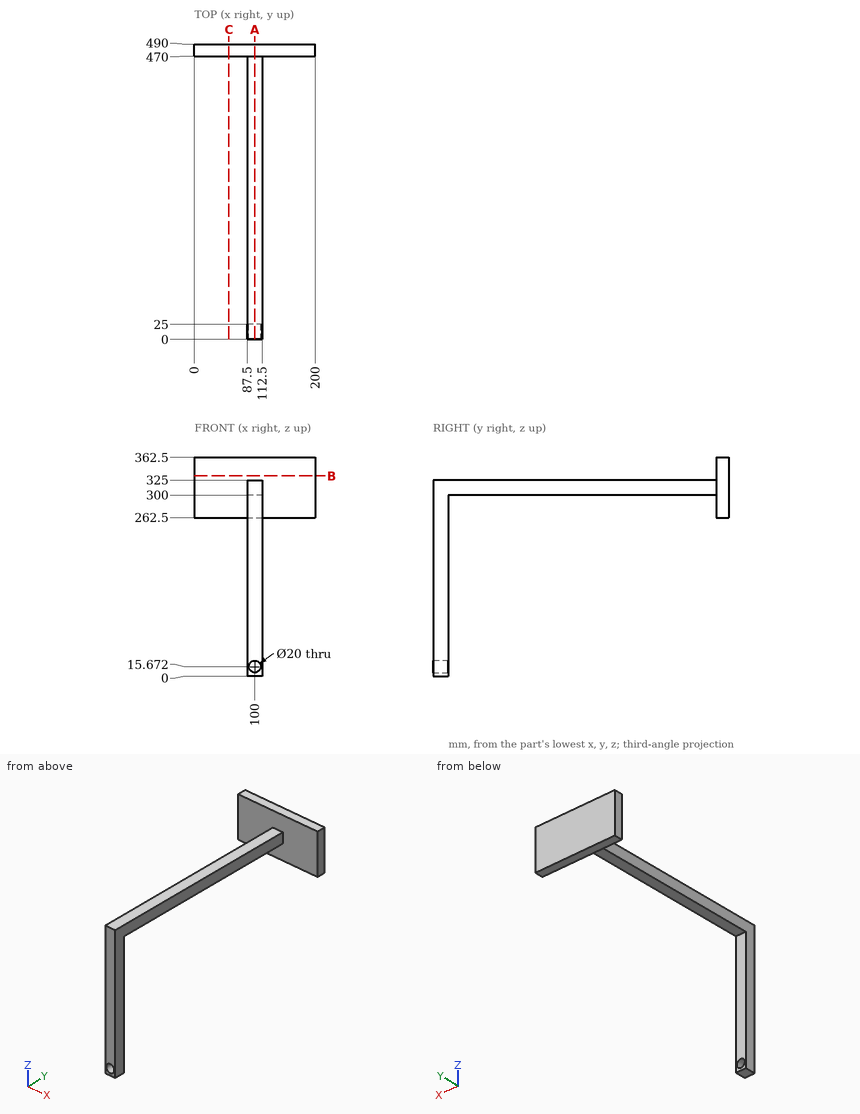
Geometry: see drawing. Coordinates: mm, zero at the bounding-box minimum. Coordinates: 2 decimals unless noted, no trailing zeros. Loops run counter-clockwise (first coordinate to the right, second up) from the corner with the lowest first, then second, coordinate; pieces in that order, holes last. Notation, with made-up numbers: (12.25, 46) -> (55.25, 46) arc R23 cw to (55.25, 82) -> close; hole circle Ø11 at (-31, 49). An arc over 180 degrees is marked (long way). Use a Markdown table: item, result.
1) Cut plane B-B (z = 332). Return the cut outline in (x, y), then the cut area to 3 significant figures.
Results found:
| item | result |
|---|---|
| outline | (0, 470) -> (200, 470) -> (200, 490) -> (0, 490) -> close |
| area | 4,000 mm2 |
2) Cut plane A-A (x = 100). Return the cut outline in (y, z), then the cut area to 4 significant figures.
Results found:
| item | result |
|---|---|
| outline | (0, 0) -> (25, 0) -> (25, 5.67) -> (0, 5.67) -> close; (0, 25.67) -> (25, 25.67) -> (25, 300) -> (470, 300) -> (470, 262.5) -> (490, 262.5) -> (490, 362.5) -> (470, 362.5) -> (470, 325) -> (0, 325) -> close |
| area | 20,750 mm2 |
3) Cut plane C-C (x = 57). Return the cut outline in (y, z).
Results found:
| item | result |
|---|---|
| outline | (470, 262.5) -> (490, 262.5) -> (490, 362.5) -> (470, 362.5) -> close |
4) Material intervals for line 1 along Y through (x, z) = (105.5, 338); line 2 along X through (y, z) = (136, 315); line 3 along Y through (x, z) = (88, 218), sorted ascending. Write a range as from..to.
Results found:
| item | result |
|---|---|
| line 1 | y = 470..490 |
| line 2 | x = 87.5..112.5 |
| line 3 | y = 0..25 |
5) Contact query for flat-ended pins moving along their axis: pin 1 (10 mm diameter, centred on x = 136, y = 478.5, fed in from -Z); pin 2 (5 mm diameter, centred on x = 107, z = 214, fed in from +Y); pin 3 (20 mm diameter, centred on x = 98.5, y = 204, fed in from +Z). Output: stop coordinate, or through.
Results found:
| item | result |
|---|---|
| pin 1 | stops at z = 262.5 |
| pin 2 | stops at y = 25 |
| pin 3 | stops at z = 325 |
